Could you check a few things on this model? Use its own coordinates, in mm. A direction names the side the tool comes from. Coordinates: 2 decimals unless noted, no trailing zeros. Order: outer loops, then holes, each group sorted by start corner. A loop starts at its lowest first (then second) coordinate and runs counter-clockwise, first axis right, second up. Notation, with made-up numbers: (75, 58.25) -> (94, 58.25) arc R16 cw to (94, 65.25) -> close; hole circle Ø8 at (64.25, 47). An arc over 180 degrees is marked (long way). Return JSON: item names as keys, results as strings. Group by question number.
from build123d import *

# Parameters (mm, degrees)
SKETCH_1_R          = 12
EXTRUDE_1_DEPTH     = 1.5
SKETCH_2_R          = 10
EXTRUDE_2_DEPTH     = 7
SKETCH_3_R          = 2
CUT_EXTRUDE_1_DEPTH = 27
SKETCH_4_R          = 4
CUT_EXTRUDE_2_DEPTH = 4


with BuildPart() as part:
    # 草图1 → 凸台-拉伸1 (new body)
    with BuildSketch(Plane.XY):
        Circle(SKETCH_1_R)
    extrude(amount=EXTRUDE_1_DEPTH)

    # 草图2 → 凸台-拉伸2 (add)
    with BuildSketch(Plane.XY.offset(1.5)):
        Circle(SKETCH_2_R)
    extrude(amount=EXTRUDE_2_DEPTH)

    # 草图3 → 切除-拉伸1 (cut)
    with BuildSketch(Plane(origin=(0, 0, 0), x_dir=(-1, 0, 0), z_dir=(0, 0, -1))):
        Circle(SKETCH_3_R)
    extrude(amount=-CUT_EXTRUDE_1_DEPTH, mode=Mode.SUBTRACT)

    # 草图4 → 切除-拉伸2 (cut)
    with BuildSketch(Plane.XY.offset(8.5)):
        Circle(SKETCH_4_R)
    extrude(amount=-CUT_EXTRUDE_2_DEPTH, mode=Mode.SUBTRACT)


solid = part.part
Q1. On a 3-axis mill with a long thin cutter (end or side, diameter ignored), from which of +Z, -Z, +X, -X, +Y, -Y can I reach the whole of each face in a straight line? I mean faces 1 (the flat face through (-5, 9, 1.5)), 2 (the cylindrical face through (-11.99, 0.53, 0.74)). Say none if no direction works.
Q2. We'd pull the mould along Y, two halves only. Please class faces 3 (the flat face through (-0.1, -4.3, 8.5)), 4 (the cylindrical face through (-2.17, -9.76, 4.95)), 5 (the cylindrical face through (-0.867, -3.905, 6.528)): pulls with the +Y half, pulls with the -Y half, needs draft (parallel to the pull), parting line crosses it, or undercut.
Q3. I want a section at C-C on z = 7.75. Please give me the cut outline in (x, y).
Q4. I need wall thicknesses on line 1 along Y through (x, z) = (0, 6.65); line 2 along Y through (x, z) = (0, 2.3); line 3 along X through (y, z) = (-3.25, 8). Which ranges of each line are inside material? Lowest first, please. Write a range as from..to.
Q5. I'm going to push flat-ended pins straight in: pin 1 Ø1.5 at (x, z) = (-5, 3.5) entering from +Y; pin 2 Ø9 at (x, y) = (1, -2) entering from +Z; pin 3 Ø1.5 at (y, z) = (-1, 6) entering from +X; pin 4 Ø1 at (y, z) = (6.5, 4.5) entering from +X. Where does each tip first touch, or does it pass through?
Q6. I want a section at D-D on y = -8.25. Please give me the cut outline in (x, z).
Q7. I want a section at A-A on y = 0. Please give me the cut outline in (x, z).
Response values:
{
 "1": {"face 1": "+Z", "face 2": "+Z, -Z"},
 "2": {"face 3": "needs draft", "face 4": "parting line crosses it", "face 5": "undercut"},
 "3": {"outline": "circle Ø20 at (0, 0); hole circle Ø8 at (0, 0)"},
 "4": {"line 1": "y = -10..-4, 4..10", "line 2": "y = -10..-2, 2..10", "line 3": "x = -9.46..-2.33, 2.33..9.46"},
 "5": {"pin 1": "stops at y = 9.05", "pin 2": "stops at z = 8.5", "pin 3": "stops at x = 10", "pin 4": "stops at x = 8"},
 "6": {"outline": "(-8.71, 0) -> (8.71, 0) -> (8.71, 1.5) -> (5.65, 1.5) -> (5.65, 8.5) -> (-5.65, 8.5) -> (-5.65, 1.5) -> (-8.71, 1.5) -> close"},
 "7": {"outline": "(-12, 0) -> (-2, 0) -> (-2, 4.5) -> (-4, 4.5) -> (-4, 8.5) -> (-10, 8.5) -> (-10, 1.5) -> (-12, 1.5) -> close; (2, 0) -> (12, 0) -> (12, 1.5) -> (10, 1.5) -> (10, 8.5) -> (4, 8.5) -> (4, 4.5) -> (2, 4.5) -> close"}
}
